The model under review builds one solid part; all positions refer to its coordinate system, in mm. Face numbers are marked on the shaded views. A direction names the side the tool comes from. Give positions to 0.01 mm unless a question says otherwise; leave off trailing zeros. Order: outer loops, then holes, each group sorted by start corner. A loop starts at its lowest first (then second) coordinate and runs counter-clockwise, first axis right, second up.
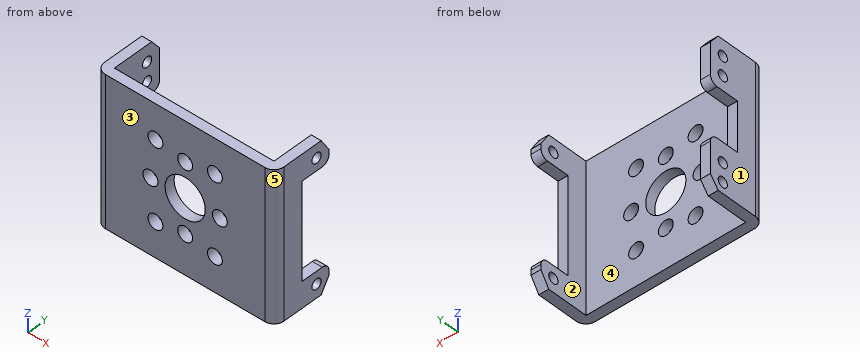
```python
from build123d import *

# Parameters (mm, degrees)
EXTRUDE_1_DEPTH     = 30
SKETCH_2_R          = 1.025
CUT_EXTRUDE_1_DEPTH = 4
SKETCH_3_R          = 1.025
CUT_EXTRUDE_2_DEPTH = 4
SKETCH_4_R          = 4.05
SKETCH_4_R_2        = 1.5
CUT_EXTRUDE_3_DEPTH = 10


with BuildPart() as part:
    # 草图1 → 凸台-拉伸1 (new body)
    with BuildSketch(Plane.XY):
        with BuildLine():
            Line((-16.1, 0), (16.1, 0))
            Line((16.1, 0), (16.1, 10))
            Line((16.1, 10), (18.1, 10))
            Line((18.1, 10), (18.1, 0))
            ThreePointArc((18.1, 0), (17.514213562, -1.414213562), (16.1, -2))
            Line((16.1, -2), (-16.1, -2))
            ThreePointArc((-16.1, -2), (-17.514213562, -1.414213562), (-18.1, 0))
            Line((-18.1, 0), (-18.1, 10))
            Line((-18.1, 10), (-16.1, 10))
            Line((-16.1, 10), (-16.1, 0))
        make_face()
    extrude(amount=EXTRUDE_1_DEPTH)

    # 草图2 → 切除-拉伸1 (cut)
    with BuildSketch(Plane(origin=(18.1, 0, 0), x_dir=(0, 0, -1), z_dir=(1, 0, 0))):
        Polygon((-30, 8.275), (-27.25, 10), (-30, 10), align=None)
        with BuildLine():
            ThreePointArc((-5.25, 8.5), (-4.810660172, 9.560660172), (-3.75, 10))
            Line((-3.75, 10), (-26.25, 10))
            ThreePointArc((-26.25, 10), (-25.189339828, 9.560660172), (-24.75, 8.5))
            Line((-24.75, 8.5), (-24.75, 4))
            Line((-24.75, 4), (-5.25, 4))
            Line((-5.25, 4), (-5.25, 8.5))
        make_face()
        with Locations((-27.25, 7.25)):
            Circle(SKETCH_2_R)
        with Locations((-2.75, 7.25)):
            Circle(SKETCH_2_R)
        Polygon((0, 10), (-2.75, 10), (0, 8.275), align=None)
    extrude(amount=-CUT_EXTRUDE_1_DEPTH, mode=Mode.SUBTRACT)

    # 草图3 → 切除-拉伸2 (cut)
    with BuildSketch(Plane.ZY.offset(18.1)):
        Polygon((0, 8.275), (2.2, 10), (0, 10), align=None)
        with Locations((2.2, 7.25)):
            Circle(SKETCH_3_R)
        with Locations((6, 7.25)):
            Circle(SKETCH_3_R)
        with BuildLine():
            Line((10, 8.5), (10, 4))
            Line((10, 4), (20, 4))
            Line((20, 4), (20, 8.5))
            ThreePointArc((20, 8.5), (20.439339828, 9.560660172), (21.5, 10))
            Line((21.5, 10), (8.5, 10))
            ThreePointArc((8.5, 10), (9.560660172, 9.560660172), (10, 8.5))
        make_face()
        with Locations((22.9, 7.25)):
            Circle(SKETCH_3_R)
        with Locations((26.7, 7.25)):
            Circle(SKETCH_3_R)
        Polygon((30, 10), (27.8, 10), (30, 8.275), align=None)
    extrude(amount=-CUT_EXTRUDE_2_DEPTH, mode=Mode.SUBTRACT)

    # 草图4 → 切除-拉伸3 (cut)
    with BuildSketch(Plane.XZ.offset(2)):
        with Locations(Location((0, 15, 0), (0, 0, 270))):
            Circle(SKETCH_4_R)
        with Locations(Location((7, 15, 0), (0, 0, 270))):
            Circle(SKETCH_4_R_2)
        with Locations(Location((0, 8, 0), (0, 0, 270))):
            Circle(SKETCH_4_R_2)
        with Locations(Location((-7, 15, 0), (0, 0, 270))):
            Circle(SKETCH_4_R_2)
        with Locations(Location((0, 22, 0), (0, 0, 270))):
            Circle(SKETCH_4_R_2)
        with Locations(Location((-6, 23.000374583, 0), (0, 0, 270))):
            Circle(SKETCH_4_R_2)
        with Locations(Location((6, 23.000374583, 0), (0, 0, 270))):
            Circle(SKETCH_4_R_2)
        with Locations(Location((-6, 7.000374583, 0), (0, 0, 270))):
            Circle(SKETCH_4_R_2)
        with Locations(Location((6, 7.000374583, 0), (0, 0, 270))):
            Circle(SKETCH_4_R_2)
    extrude(amount=-CUT_EXTRUDE_3_DEPTH, mode=Mode.SUBTRACT)


solid = part.part
```
Item 1: Take a section at C-C (y = 5.5). Give the boundary of the cut face in (x, z), and give its area (3 significant figures).
Values found:
outline: (-18.1, 0) - (-16.1, 0) - (-16.1, 10) - (-18.1, 10) - close; (-18.1, 20) - (-16.1, 20) - (-16.1, 30) - (-18.1, 30) - close; (16.1, 0) - (18.1, 0) - (18.1, 5.25) - (16.1, 5.25) - close; (16.1, 24.75) - (18.1, 24.75) - (18.1, 30) - (16.1, 30) - close
area: 61.0 mm2
Item 2: Take a section at B-B (y = 0.5). Give the boundary of the cut face in (x, z), and give its area (3 significant figures).
Values found:
outline: (-18.1, 0) - (-16.1, 0) - (-16.1, 30) - (-18.1, 30) - close; (16.1, 0) - (18.1, 0) - (18.1, 30) - (16.1, 30) - close
area: 120 mm2
Item 3: Take a section at D-D (x = 3). Give the boundary of the cut face in (y, z), and give its area (3 significant figures).
Values found:
outline: (-2, 0) - (0, 0) - (0, 12.28) - (-2, 12.28) - close; (-2, 17.72) - (0, 17.72) - (0, 30) - (-2, 30) - close
area: 49.1 mm2
Item 4: For line 1 (X direction, y = 0.75, z = 10.75); line 2 (Y direction, x = 15, z = 16.75); line 3 (X direction, y = 7.5, z = 7.75), list the stretches that pass through material, from the lowest coordinate up.
Values found:
line 1: x = -18.1 to -16.1, 16.1 to 18.1
line 2: y = -2 to 0
line 3: x = -18.1 to -16.1
Item 5: Draft analysis for pull direction X (two halves, no side actions). For the marked faces 1, 2 and 3, state which applies: released by +X, released by -X, zero draft, split by the parting line, or undercut.
Values found:
face 1: released by -X
face 2: undercut
face 3: zero draft
Item 6: Take a section at A-A (z = 15). Give the boundary of the cut face in (x, y), and give its area (3 significant figures).
Values found:
outline: (-18.1, 0) arc R2 ccw to (-16.1, -2) - (-8.5, -2) - (-8.5, 0) - (-16.1, 0) - (-16.1, 4) - (-18.1, 4) - close; (-5.5, -2) - (-4.05, -2) - (-4.05, 0) - (-5.5, 0) - close; (4.05, -2) - (5.5, -2) - (5.5, 0) - (4.05, 0) - close; (8.5, -2) - (16.1, -2) arc R2 ccw to (18.1, 0) - (18.1, 4) - (16.1, 4) - (16.1, 0) - (8.5, 0) - close
area: 58.5 mm2
Item 7: Clearance check with flat-ended pins moving along their axes: pin 1 Ø10 at (x, z) = (0.5, 25) entering from +Y; pin 2 Ø5 at (x, z) = (0, 15) entering from -Y; pin 3 Ø1.6 at (x, z) = (17.5, 13) entering from +Y; pin 4 Ø1.6 at (y, z) = (7.25, 6) entering from -X. State where each tip first meets the part, or that it passes through.
Values found:
pin 1: stops at y = 0
pin 2: passes through
pin 3: stops at y = 4
pin 4: stops at x = 16.1
Item 8: For the marked faces 4 and 5, list the 3-axis set-ups (+Z, -Z, +X, -X, +Y, -Y) from which the entire face can be reached by the end or side of a thin tool; tool diameter is ignored.
Values found:
face 4: +Z, -Z, +Y
face 5: +Z, -Z, +X, -Y
